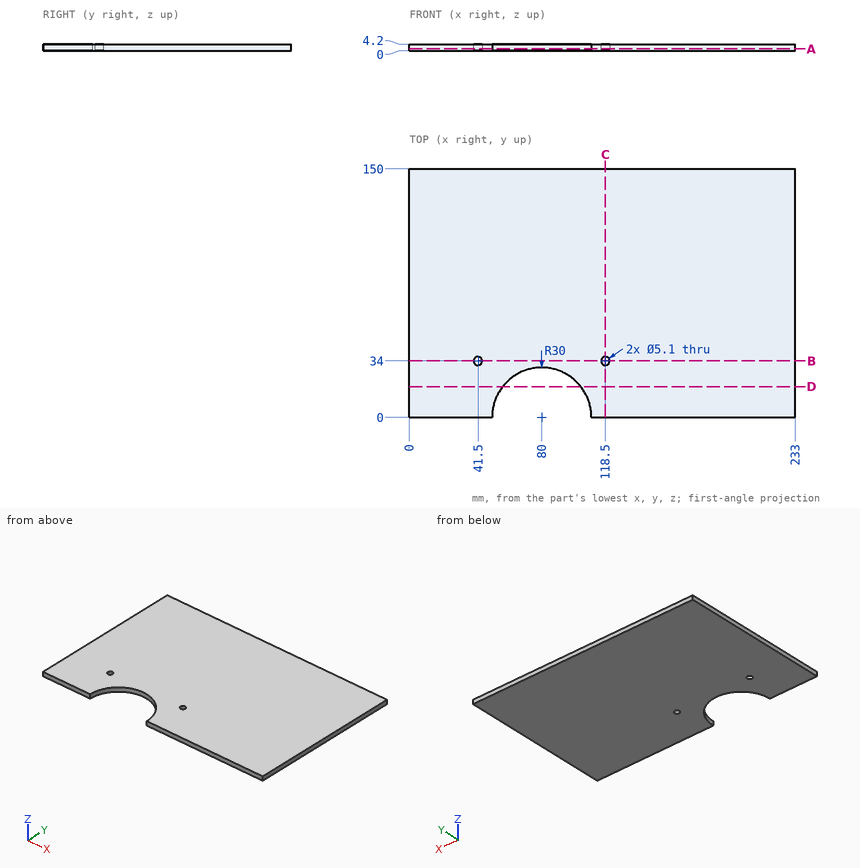
Study the drawing (mm; zero at the part's minimum x, y, z) and answer. Give positions to 0.01 mm unless a question says otherwise; leave off trailing zeros. Write each loop counter-clockwise with the first axis right and the second up, starting at its lowest first coordinate (ties: lowest second). Pieces come first, ordered by that corner, then holes.
Item 1: Find the intervals of material crossed by line 1 along Y through (x, z) = (118.5, 3.35); line 2 along X through (y, z) = (23.5, 0.35); line 3 along X through (y, z) = (16, 0.9), in increasing order.
Item 2: Section D-D, the plane y = 18.5 is taken. Write down the section's boundary in (x, z), plus the area to 3 significant figures.
Item 3: Section A-A, the plane z = 1.25 is taken. Write down the section's boundary in (x, y), plus the area to 3 significant figures.
Item 4: Section B-B, the plane y = 34 is taken. Write down the section's boundary in (x, z), plus the area to 3 significant figures.
Item 5: Section C-C, the plane x = 118.5 is taken. Write down the section's boundary in (y, z), plus the area to 3 significant figures.
Item 6: A flat-ended cylindrical pin translates along its axis: P1, Ø1.5, axis at x = 71, z = 3, coming from the -Y side. Find the tip coordinate at first contact, or state that the pin passes through.
Completed:
1. line 1: y = 0 to 31.45, 36.55 to 150
1. line 2: x = 0 to 61.35, 98.65 to 233
1. line 3: x = 0 to 54.62, 105.38 to 233
2. outline: (0, 0) - (56.38, 0) - (56.38, 4.2) - (0, 4.2) - close; (103.62, 0) - (233, 0) - (233, 4.2) - (103.62, 4.2) - close
2. area: 780 mm2
3. outline: (0, 0) - (50, 0) arc R30 cw to (110, 0) - (233, 0) - (233, 150) - (0, 150) - close; hole circle Ø5.1 at (41.5, 34); hole circle Ø5.1 at (118.5, 34)
3. area: 33,500 mm2
4. outline: (0, 0) - (38.95, 0) - (38.95, 4.2) - (0, 4.2) - close; (44.05, 0) - (115.95, 0) - (115.95, 4.2) - (44.05, 4.2) - close; (121.05, 0) - (233, 0) - (233, 4.2) - (121.05, 4.2) - close
4. area: 936 mm2
5. outline: (0, 0) - (31.45, 0) - (31.45, 4.2) - (0, 4.2) - close; (36.55, 0) - (150, 0) - (150, 4.2) - (36.55, 4.2) - close
5. area: 609 mm2
6. P1: stops at y = 28.37
